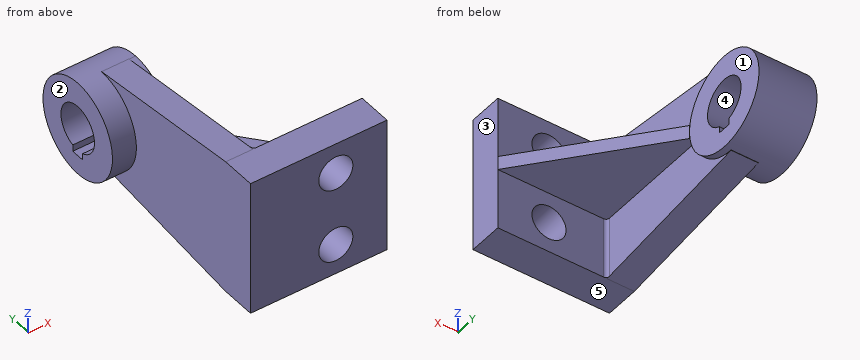
Autodesk Inventor part; units mm, degrees
ref_plane "YZ Plane" through (0, 0, 0) normal (1, 0, 0) x (0, 1, 0)
ref_plane "XZ Plane" through (0, 0, 0) normal (0, 1, 0) x (-1, 0, 0)
ref_plane "XY Plane" through (0, 0, 0) normal (0, 0, 1) x (1, 0, 0)
sketch "Boceto2" plane through (0, 0, 0) normal (0, 1, 0) x (-1, 0, 0)
  line L0 (0, 0) -> (0, 40) construction
  line L1 (0, 40) -> (-47, 40)
  line L2 (-47, 40) -> (-47, 0)
  line L3 (-47, 0) -> (-47, -40)
  line L4 (-47, 0) -> (-17, 0) construction
  line L5 (-17, 0) -> (-17, -22) construction
  circle A0 centre (-17, -22) radius 10
  line L6 (-17, 0) -> (-17, 22) construction
  circle A1 centre (-17, 22) radius 10
  line L7 (-47, 0) -> (-47, -4) construction
  line L8 (-47, -4) -> (13, -4)
  line L9 (-47, 0) -> (-47, 4) construction
  line L10 (17, 40) -> (17, 28)
  line L11 (17, -28) -> (17, -40)
  line L12 (33, -40) -> (33, -28)
  line L13 (-47, -40) -> (0, -40)
  line L14 (0, -40) -> (17, -40)
  line L15 (33, -40) -> (17, -40)
  line L16 (0, 40) -> (17, 40)
  line L17 (33, 28) -> (33, 40)
  line L18 (47, 40) -> (33, 40) construction
  line L19 (33, 40) -> (17, 40)
  line L20 (13, -40) -> (47, -40) construction
  line L21 (33, 28) -> (33, -28)
  line L22 (17, 28) -> (17, -28)
  line L23 (-47, 4) -> (17, 4)
  line L24 (13, -4) -> (17, -4)
  line L25 (47, -40) -> (47, 40) construction
  line L26 (-47, 0) -> (17, 0)
  dimension "d2" = 40
  dimension "d4" = 47
  dimension "d5" = 40
  dimension "d10" = 30
  dimension "d11" = 22
  dimension "d12" = 20
  dimension "d16" = 4
  dimension "d17" = 4
  dimension "d41" = 16
  dimension "d44" = 34
extrude "Extrusión5" add sketch "Boceto2" along normal blind 20 contours L16 L10 L22 L23 L2 L1 | L8 L24 L22 L11 L14 L13 L3
extrude "Extrusión8" add sketch "Boceto2" along normal blind 120 contours L19 L17 L21 L12 L15 L11 L22 L10
sketch "Boceto12" plane through (-33, 0, -40) normal (-1, 0, 0) x (0, 0, 1)
  line L0 (0, 20) -> (0, 120)
  line L1 (0, 0) -> (0, 20)
  line L2 (80, 0) -> (80, 20)
  line L3 (0, 20) -> (80, 20)
  line L4 (80, 20) -> (80, 0)
  line L5 (80, 0) -> (0, 0)
  line L6 (40, 0) -> (40, 120) construction
  circle A0 centre (40, 120) radius 28
  arc A1 (27.1062, 116) -> (27.1062, 124) centre (40, 120) ccw
  line L7 (12.1931, 123.2828) -> (0, 20)
  line L8 (67.8069, 123.2828) -> (80, 20)
  line L9 (0, 120) -> (80, 120)
  line L10 (53.5, 120) -> (23.2, 120) construction
  line L11 (23.2, 120) -> (23.2, 124)
  line L12 (23.2, 124) -> (27.1062, 124)
  line L13 (23.2, 120) -> (23.2, 116)
  line L14 (23.2, 116) -> (27.1062, 116)
  line L15 (80, 120) -> (0, 120)
  line L16 (80, 120) -> (80, 22.7295)
  line L17 (80, 20) -> (80, 120)
  point P0 (68, 120)
  point P1 (68.1944, 120)
  point P2 (11.8056, 120)
  dimension "d68" = 56
  dimension "d69" = 27
  dimension "d70" = 30.3
extrude "Extrusión9" add sketch "Boceto12" along normal blind 14 and the other way blind 20 contours A0 L9 A1 L12 L11 | L9 L13 L14 A1 A0
extrude "Extrusión10" cut sketch "Boceto12" against normal blind 30 contours L0 L9 L7 | L8 L9 L16 L17 | L9 A1 L14 L13
extrude "Extrusión13" add sketch "Boceto2" along normal blind 92 contours L23 L22 L26 L2 | L26 L22 L24 L8 L3
sketch "Boceto15" plane through (-17, 20, 4) normal (0, 0, 1) x (1, 0, 0)
  arc A0 (-16, 70) -> (-18, 72) centre (-18, 70) ccw
  arc A1 (0, 2) -> (2, 0) centre (2, 2) ccw
  arc A2 (2, 72) -> (0, 70) centre (2, 70) ccw
  line L0 (0, 72) -> (64, 72)
  line L1 (0, 100) -> (0, 0)
  line L2 (-16, 0) -> (-16, 100)
  line L3 (-30, 128) -> (-30, 72)
  line L4 (-30, 72) -> (-16, 72)
  line L5 (0, 0) -> (64, 0)
  line L6 (64, 72) -> (0, 72)
  line L7 (0, 72) -> (4, 72)
  line L8 (4, 72) -> (64, 0)
  line L9 (4, 72) -> (64, 72)
  line L10 (64, 72) -> (64, 0)
  point P0 (17, -20)
  point P1 (4, 72)
  dimension "d90" = 4
  dimension "d92" = 4
  dimension "d93" = 4
  dimension "d94" = 4
extrude "Extrusión14" cut sketch "Boceto15" against normal blind 20 contours L8 L0 L10
extrude "Extrusión15" add sketch "Boceto15" along normal blind 36 and the other way blind 44 contours A1 L5 L1
properties part number "Soporte_Tensor" material "Iron, Malleable"
Work out the finished part from the listing and answer in its coordinate system (mm). Face numbers are marked on the shaded views. A direction names the side the tool comes from. Coordinates: 2 decimals unless noted, no trailing zeros. Write each loop counter-clockwise with the first axis right and the second up, starting at its lowest first coordinate (ties: lowest second). Pieces come first, ordered by that corner, then holes. Notation, with made-up numbers: (4.25, 50) - (40.25, 50) arc R15 ccw to (40.25, 54) - close; hole circle Ø3 at (89.25, 41). An arc over 180 degrees is marked (long way). Answer as a JSON object with one key per item and string values.
Q1. Find section D-D (y = 50). Write down the section's boundary in (x, z), plus the area to 3 significant figures.
Results list:
{"outline": "(-33, -36.46) - (-17, -36.46) - (-17, -4) - (22, -4) - (22, 4) - (-17, 4) - (-17, 36.46) - (-33, 36.46) - close", "area": "1,480 mm^2"}
Q2. Find section A-A (x = 17). Write down the section's boundary in (y, z), plus the area to 3 significant figures.
Results list:
{"outline": "(0, -40) - (20, -40) - (20, -32) - (0, -32) - close; (0, -12) - (20, -12) - (20, -4) - (56, -4) - (56, 4) - (20, 4) - (20, 12) - (0, 12) - close; (0, 32) - (20, 32) - (20, 40) - (0, 40) - close", "area": "1,090 mm^2"}
Q3. Which of the six approach directions +Z, -Z, +X, -X, +Y, -Y give full straight-line access (tool end or side, diameter ignored) to the marked faces 1 and 2?
Results list:
{"face 1": "+Z, -Z, +X, +Y", "face 2": "+Z, -Z, -X, +Y, -Y"}
Q4. Given pin 1 Ø4 at (x, y) = (17, 56) entering from -Z; pin 2 Ø12 at (y, z) = (126.5, 5.5) entering from +X; pin 3 Ø8 at (x, y) = (33.5, 46) entering from +Z; pin 4 Ø3 at (y, z) = (75.5, 22) entering from -X, each flat-ended and moving along its own axis, determine where each tip first touches the part or whether it passes through.
Results list:
{"pin 1": "stops at z = -4", "pin 2": "stops at x = -13", "pin 3": "passes through", "pin 4": "stops at x = -33"}
Q5. Find section B-B (z = 22). Write down the section's boundary in (x, y), plus the area to 3 significant figures.
Results list:
{"outline": "(-47, 102.68) - (-33, 102.68) - (-33, 0) - (7, 0) - (7, 20) - (-15, 20) arc R2 cw to (-17, 22) - (-17, 102.68) - (-13, 102.68) - (-13, 137.32) - (-47, 137.32) - close; (27, 0) - (47, 0) - (47, 20) - (27, 20) - close", "area": "3,700 mm^2"}
Q6. Consider L1, parallel to Z at x = 17, y = 14; L2, parallel to Z at x = -38, y = 120; L3, parallel to X at y = 23, z = 36.5. Determine where each line is inside the solid, lowest interval first. Write a range as from..to.
Results list:
{"L1": "z = -40..-32, -12..12, 32..40", "L2": "z = -28..-16.8, 13.5..28", "L3": "x = -33..-17"}
Q7. Find section C-C (x = -1.5). Write down the section's boundary in (y, z), plus the area to 3 significant figures.
Results list:
{"outline": "(0, -40) - (20, -40) - (20, -4) - (78.2, -4) - (78.2, 4) - (20, 4) - (20, 40) - (0, 40) - close", "area": "2,070 mm^2"}
Q8. For a pull along Z with two mould halves and no side action, classify the marked faces 3, 4 and 5 as pulls with the +Z half, pulls with the -Z half, needs draft (parallel to the pull), parting line crosses it, or undercut.
Results list:
{"face 3": "needs draft", "face 4": "undercut", "face 5": "pulls with the -Z half"}
